Print and shaded views of the part. All mm, measured from the part's lowest x, y and z. A direction names the side the tool comes from. Round coordinates to 2 decimals unless told otherwise and drop trailing zeros. Order: outer loops, then holes, each group sorted by start corner. A loop starts at its lowest first (then second) coordinate and runs counter-clockwise, first axis right, second up.
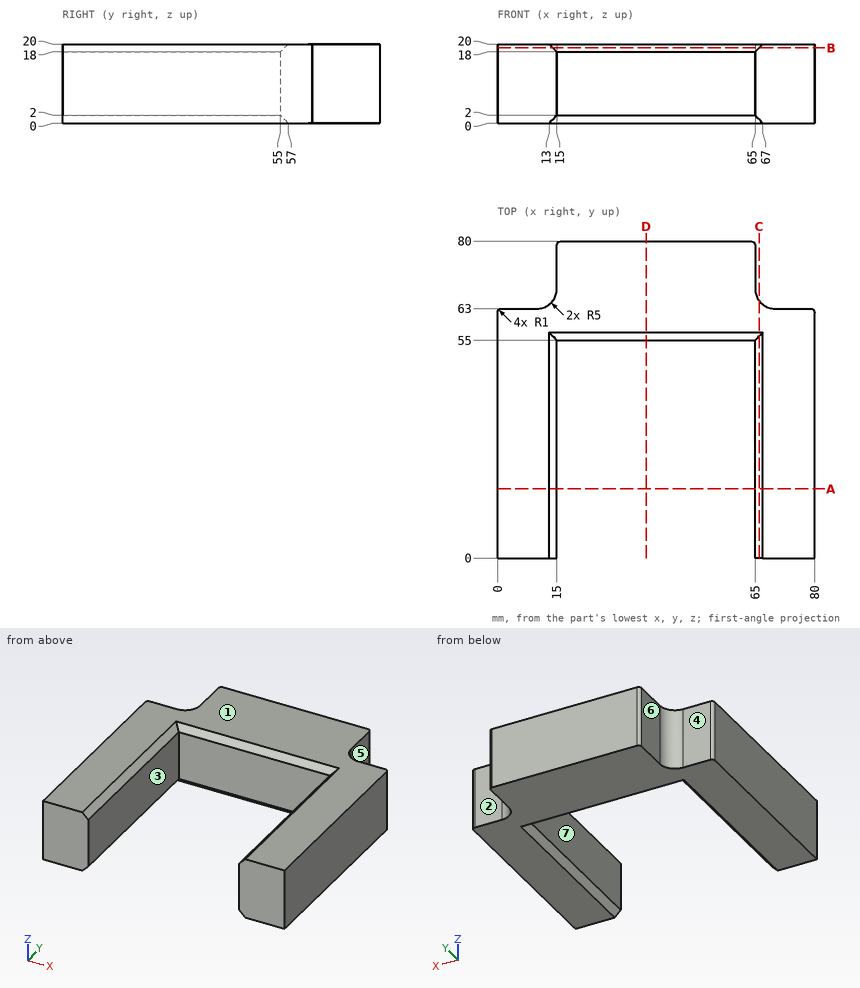
1. Cut at D-D, the plane x = 37.5. Write the cut outline in (y, z).
2. Cut at C-C, the plane x = 66. Write the cut outline in (y, z), and give its area (3 significant figures).
3. Pin check, flat tips, straight feed: P1, Ø3.5, axis at y = 74.5, z = 8.5, coming from the +X side; P2, Ø4, axis at x = 61, z = 3, coming from the -Y side; P3, Ø5, axis at y = 17, z = 6.5, coming from the -X side; P4, Ø10, axis at x = 6, z = 6, coming from the +Y side. Stop position of each tip, or through.
4. Cut at B-B, the plane z = 19. Write the cut outline in (x, y), and give its area (3 significant figures).
5. Mould opens along X. For the marked faces 5, 6 and 7 say: released by +X, released by -X, zero draft, split by the parting line, or undercut.
6. Tool access for the marked faces 1, 2, 3 and 4: list every direction of +Z, -Z, +X, -X, +Y, -Y with a clear straight run to the whole face (end or side of a thin tool).
7. Drill centre lines: line 1 (X direction, y = 6.5, z = 5.75); line 2 (Y direction, x = 66, z = 3.5); line 3 (Y direction, x = 54, z = 17). Where is each one in solid material? Low to high.
8. Cut at A-A, the plane y = 17.5. Write the cut outline in (x, z), and give its area (3 significant figures).
Outcome:
1. outline: (55, 2) - (57, 0) - (80, 0) - (80, 20) - (57, 20) - (55, 18) - close
2. outline: (0, 1) - (56, 1) - (57, 0) - (65, 0) - (65, 20) - (57, 20) - (56, 19) - (0, 19) - close
2. area: 1,190 mm2
3. P1: stops at x = 65
3. P2: stops at y = 55
3. P3: stops at x = 0
3. P4: stops at y = 63.1
4. outline: (0, 0) - (14, 0) - (14, 56) - (66, 56) - (66, 0) - (80, 0) - (80, 62) arc R1 ccw to (79, 63) - (70, 63) arc R5 cw to (65, 68) - (65, 79) arc R1 ccw to (64, 80) - (16, 80) arc R1 ccw to (15, 79) - (15, 68) arc R5 cw to (10, 63) - (1, 63) arc R1 ccw to (0, 62) - close
4. area: 2,990 mm2
5. face 5: released by +X
5. face 6: released by -X
5. face 7: undercut
6. face 1: +Z, +X, -X, +Y, -Y
6. face 2: +Z, -Z, +X, +Y
6. face 3: +Z, -Z, -Y
6. face 4: +Z, -Z, -X, +Y
7. line 1: x = 0 to 15, 65 to 80
7. line 2: y = 0 to 65
7. line 3: y = 55 to 80
8. outline: (0, 0) - (13, 0) - (15, 2) - (15, 18) - (13, 20) - (0, 20) - close; (65, 2) - (67, 0) - (80, 0) - (80, 20) - (67, 20) - (65, 18) - close
8. area: 592 mm2
